Build history of the part. All positions in model axes, mm. Coordinates: 2 decimals unless noted, no trailing zeros. Write each loop counter-clockwise with the first axis right and the second up, starting at its lowest first coordinate (ties: lowest second). Pieces come first, ordered by that corner, then holes. Notation, with made-up numbers: (17.5, -37.5) -> (55.5, -37.5) arc R25 cw to (55.5, -14.5) -> close; hole circle Ø1 at (61, -17.75). An arc over 180 degrees is marked (long way). Write each question's results on one line, items separated by ' | '. Start each with the question number.
Q1. Drop flat-ended pins along their axis: pin 1 Ø2.5 at (x, y) = (-13.27, 22.98) entering from +Z; pin 2 Ø1.5 at (y, z) = (-19.5, 2.5) entering from -X; pin 3 Ø3 at (x, y) = (20, -11.5) entering from -Z. Give the stop position or say it passes through.
Q2. Saw through at C-C on x = 18.5. Give the cut face in (y, z), and give its area (3 significant figures).
Q3. Saw through at B-B on y = 9.5. Give the cut face in (x, z), and give its area (3 significant figures).
Q4. Saw through at A-A on z = 1.3. Give the cut face in (x, y).
Q5. Two-plate mould, pull along X, no slides. Class faces 1 (the face through (14.07, -24.25, 1.48)), 2 (the face through (0, 0, 3)), 3 (the face through (22.395, -13.172, 1.479)): released by +X, released by -X, zero draft, split by the parting line, or undercut.
Q6. Drill centre lines: line 1 (X direction, y = 23, z = 1); line 2 (Y direction, x = -23.5, z = 0.8); line 3 (Y direction, x = -25.5, z = 2.6). Where is each one in solid material? Low to high.
Autodesk Inventor part; units mm, degrees
ref_plane "YZ Plane" through (0, 0, 0) normal (1, 0, 0) x (0, 1, 0)
ref_plane "XZ Plane" through (0, 0, 0) normal (0, 1, 0) x (-1, 0, 0)
ref_plane "XY Plane" through (0, 0, 0) normal (0, 0, 1) x (1, 0, 0)
sketch "Sketch1" plane through (0, 0, 0) normal (0, 0, 1) x (1, 0, 0)
  line L0 (-29.9999, 0.0001) -> (-15, -25.9807)
  line L1 (15, -25.9808) -> (30, 0)
  line L2 (-15, -25.9807) -> (15, -25.9808)
  line L3 (30, 0) -> (15, 25.9808)
  line L4 (15, 25.9808) -> (-15, 25.9808)
  line L5 (-15, 25.9808) -> (-30, 0)
  line L6 (0, 25.9808) -> (0, -25.9808) construction
  line L7 (-30, 0) -> (30, 0) construction
  line L8 (-24.8039, 3) -> (-13.268, 22.9808) construction
  line L9 (-13.268, 22.9808) -> (13.2679, 22.9808) construction
  line L10 (13.2679, 22.9808) -> (24.8038, 3) construction
  line L11 (24.8038, 3) -> (-24.8039, 3) construction
  circle A0 centre (-13.268, 22.9808) radius 1.5
  circle A1 centre (13.2679, 22.9808) radius 1.5
  circle A2 centre (-24.8039, 0) radius 1.5 construction
  line L12 (-24.8039, 3) -> (-26.5359, 0) construction
  circle A3 centre (24.8039, 0.0001) radius 1.5 construction
  circle A4 centre (-13.268, -22.9808) radius 1.5
  circle A5 centre (13.2679, -22.9808) radius 1.5
  point P0 (0, 0)
  point P1 (0, 0)
  point P2 (-30, 0.0001)
  dimension "d1" = 30
  dimension "d6" = 120
  dimension "d7" = 120
  dimension "d8" = 120
  dimension "d9" = 120
  dimension "d10" = 120
  dimension "d13" = 3
  dimension "d14" = 3
  dimension "d15" = 3
extrude "Extrusion1" add sketch "Sketch1" along normal blind 3
equation "\"d7\" = d6"
equation "\"d8\" = d6"
equation "\"d9\" = d6"
equation "\"d10\" = d6"
properties part number "ArmControlBoard"
Returned:
1) pin 1: passes through | pin 2: stops at x = -19.17 | pin 3: stops at z = 0
2) outline: (-19.92, 0) -> (19.92, 0) -> (19.92, 3) -> (-19.92, 3) -> close | area: 120 mm2
3) outline: (-24.52, 0) -> (24.52, 0) -> (24.52, 3) -> (-24.52, 3) -> close | area: 147 mm2
4) outline: (-30, 0) -> (-15, -25.98) -> (15, -25.98) -> (30, 0) -> (15, 25.98) -> (-15, 25.98) -> close; hole circle Ø3 at (-13.27, -22.98); hole circle Ø3 at (-13.27, 22.98); hole circle Ø3 at (13.27, -22.98); hole circle Ø3 at (13.27, 22.98)
5) face 1: undercut | face 2: zero draft | face 3: released by +X
6) line 1: x = -16.72 to -14.77, -11.77 to 11.77, 14.77 to 16.72 | line 2: y = -11.26 to 11.26 | line 3: y = -7.79 to 7.79
